from build123d import *

# Parameters (mm, degrees)
BOSS_EXTRUDE1_DEPTH = 3
BOSS_EXTRUDE3_DEPTH = 38


with BuildPart() as part:
    # Sketch1 → Boss-Extrude1 (new body)
    with BuildSketch(Plane(origin=(0, 0, 0), x_dir=(1, 0, 0), z_dir=(0, 1, 0))):
        Polygon((-35, 0), (0, 0), (0, 15), (-35, 11), align=None)
        Polygon((-35, -11), (0, -15), (0, 0), (-35, 0), align=None)
    extrude(amount=BOSS_EXTRUDE1_DEPTH)

    # Sketch2 → Boss-Extrude3 (add)
    with BuildSketch(Plane(origin=(0, 3, 0), x_dir=(1, 0, 0), z_dir=(0, 1, 0))):
        Polygon((-35, 11), (-35, -11), (0, -15), (0, -11.980471722), (-32, -8.323328865), (-32, 8.323328865), (0, 11.980471722), (0, 15), align=None)
    extrude(amount=BOSS_EXTRUDE3_DEPTH)


solid = part.part
Model file for the job. Use its own axes, mm. A direction names the side the tool comes from. Coordinates: 2 decimals unless noted, no trailing zeros. Order: outer loops, then holes, each group sorted by start corner. A loop starts at its lowest first (then second) coordinate and runs counter-clockwise, first axis right, second up. Notation, with made-up numbers: (-3, 62.5) -> (29, 62.5) arc R37 ccw to (29, 98.5) -> close; hole circle Ø7 at (6, 4). An arc over 180 degrees is marked (long way). Return JSON: item names as keys, results as strings. Group by question number.
Item 1: Wall check: line 1 along Y through (x, z) = (-12.5, -6.5); line 2 along Z through (x, y) = (-1.5, 29); line 3 along X through (y, z) = (23, -4.5). Give the ranges that are in metal, low to high. Write a range as [from, to].
Item 2: Pull direction Z, two halves, no side cores. Call faces 1 (the flat face through (0, 15.8, 12.3)), 2 (the flat face through (-32, 22, 0)), 3 (the flat face through (-17.745, 20.213, 12.972)): pulls with the +Z half, pulls with the -Z half, needs draft (parallel to the pull), parting line crosses it, or undercut.
Item 3: Tool access for faces 4 (the flat face through (-18, 0, 0)), 5 (the flat face through (-16.224, 21.734, -10.126)): list every direction of +Z, -Z, +X, -X, +Y, -Y with a clear straight run to the whole face (end or side of a thin tool).
Item 4: Saw through at B-B on x = -3. Write the cut outline in (y, z).
Item 5: Saw through at A-A on y = 17.5. Write the cut outline in (x, z), then the cut area to 3 significant figures.
Item 6: Saw through at C-C on z = 5. Write the cut outline in (x, y), then the cut area to 3 significant figures.
Item 7: Flat gauge pins, fed straight in: P1, Ø13.5, axis at y = 21, z = -0.5, coming from the +X side; P2, Ø3, axis at x = -21, y = 13.5, coming from the +Z side; P3, Ø12, axis at x = -19, z = 1, coming from the +Y side. Where does each tip first touch, or does it go through?
Item 8: Saw through at D-D on z = 12.5. Write the cut outline in (x, y) (3 decimals).
Values found:
{
 "1": {"line 1": "y = [0, 3]", "line 2": "z = [-14.83, -11.81], [11.81, 14.83]", "line 3": "x = [-35, -32]"},
 "2": {"face 1": "needs draft", "face 2": "undercut", "face 3": "pulls with the +Z half"},
 "3": {"face 4": "+Z, -Z, +X, -X, -Y", "face 5": "+X, +Y"},
 "4": {"outline": "(0, -14.66) -> (41, -14.66) -> (41, -11.64) -> (3, -11.64) -> (3, 11.64) -> (41, 11.64) -> (41, 14.66) -> (0, 14.66) -> close"},
 "5": {"outline": "(-35, -11) -> (0, -15) -> (0, -11.98) -> (-32, -8.32) -> (-32, 8.32) -> (0, 11.98) -> (0, 15) -> (-35, 11) -> close", "area": "260 mm2"},
 "6": {"outline": "(-35, 0) -> (0, 0) -> (0, 3) -> (-32, 3) -> (-32, 41) -> (-35, 41) -> close", "area": "219 mm2"},
 "7": {"P1": "stops at x = -32", "P2": "stops at z = 12.77", "P3": "stops at y = 3"},
 "8": {"outline": "(-21.875, 0) -> (0, 0) -> (0, 41) -> (-21.875, 41) -> close"}
}
